```python
from build123d import *

# Parameters (mm, degrees)
F1_DEPTH = 40.2336
F0_R     = 10.16
F2_DEPTH = 15.7734
F3_R     = 3.302


with BuildPart() as f1:
    # F0 (on Top) → F1 (new body)
    with BuildSketch(Plane.XY):
        with BuildLine():
            ThreePointArc((5.042647, 28.126541), (-28.575, 0), (5.042647, -28.126541))
            ThreePointArc((5.042647, -28.126541), (21.916025, -18.336262), (28.575, 0))
            ThreePointArc((28.575, 0), (21.916025, 18.336262), (5.042647, 28.126541))
        make_face()
        with BuildLine():
            ThreePointArc((13.447765, -4.826), (-14.2875, 0), (13.447765, 4.826))
            Line((13.447765, 4.826), (18.542, 4.826))
            Line((18.542, 4.826), (18.542, -4.826))
            Line((18.542, -4.826), (13.447765, -4.826))
        make_face(mode=Mode.SUBTRACT)
    extrude(amount=F1_DEPTH)

    # F0 (on Top) → F2 (join)
    with BuildSketch(Plane.XY):
        with BuildLine():
            Line((5.042647, -28.126541), (57.336765, -18.751028))
            ThreePointArc((57.336765, -18.751028), (73.025, 0), (57.336765, 18.751028))
            Line((57.336765, 18.751028), (5.042647, 28.126541))
            ThreePointArc((5.042647, 28.126541), (21.916025, 18.336262), (28.575, 0))
            ThreePointArc((28.575, 0), (21.916025, -18.336262), (5.042647, -28.126541))
        make_face()
        with Locations((53.975, 0)):
            Circle(F0_R, mode=Mode.SUBTRACT)
    extrude(amount=F2_DEPTH)

    # F3
    f3_edges = [f1.edges().sort_by_distance(p)[0] for p in [
        (-5.042647, 28.126541, 40.2336),
    ]]
    fillet(f3_edges, radius=F3_R)


solid = f1.part
```
Read the model definition and answer for the solid it produces. Units are mm, in the model's axes. A direction names the side the tool comes from. Give positions to 0.01 mm unless a question says otherwise; leave off trailing zeros. Order: outer loops, then holes, each group sorted by start corner. A loop starts at its lowest first (then second) coordinate and runs counter-clockwise, first axis right, second up. Notation, with made-up numbers: (86.25, 7) -> (107.25, 7) arc R31 cw to (107.25, 42) -> close; hole circle Ø2 at (54.5, 45.25). An arc over 180 degrees is marked (long way). Write item = value, one per line.
1. For faces 1 (the face through (31.556, 23.373, 7.776)), 2 (the face through (16, -4.826, 20)), determine the directions among +Z, -Z, +X, -X, +Y, -Y from which every point of the face is accessible in a straight line to the end or side of a thin tool.
Numbers:
face_1 = +Z, -Z, +X, +Y
face_2 = +Z, -Z
2. Straight lines are drawn through the part: line 1 along Y through (x, z) = (0, 23) (1 decimal); line 2 along X through (y, z) = (0, 24) (1 decimal); line 3 along Z through (x, y) = (39, 9.5). For each, find the intervals that lie inside material, in ascending order.
Numbers:
line_1 = -28.6 to -14.3, 14.3 to 28.6
line_2 = -28.6 to -14.3, 18.5 to 28.6
line_3 = 0 to 15.77
3. A cutting plane is placed at A-A, the plane z = 10. Count the separate pieces of the cut face and the enclosed holes in it, and give its area (3 significant figures).
Numbers:
separate_pieces = 1
enclosed_holes = 2
area = 3,450 mm²
4. The mould has two halves that part along X. Classify faces 3 (the face through (11, -11, 40.234)), 4 (the face through (30.824, -23.504, 7.776)), 5 (the face through (16, 4.826, 20)): +X half, -X half, draft (parallel to the pull), parting line (faces both ways), or undercut.
Numbers:
face_3 = draft
face_4 = +X half
face_5 = undercut
5. Given pin 1 (3 mm diameter, centred on y = -17.5, z = 4.5, fed in from +X); pin 2 (4 mm diameter, centred on x = -7, z = 35.5, fed in from -Y); pin 3 (10.5 mm diameter, centred on y = -1.5, z = 28.5, fed in from -X) (3 decimals), each flat-ended and moving along its own axis, determine where each tip first touches the part or whether it passes through.
Numbers:
pin_1 = 64.31
pin_2 = -28.13
pin_3 = -28.575
6. A cutting plane is placed at B-B, the plane x = 51. Write down the section's boundary in (y, z), and give its area (3 significant figures).
Numbers:
outline = (-19.89, 0) -> (-9.71, 0) -> (-9.71, 15.77) -> (-19.89, 15.77) -> close; (9.71, 0) -> (19.89, 0) -> (19.89, 15.77) -> (9.71, 15.77) -> close
area = 321 mm²
